from build123d import *

# Parameters (mm, degrees)
F0_W      = 609.6
F0_H      = 38.1
F1_DEPTH  = 203.2
F3_D      = 5.1054
F5_D      = 5.1054
F5_DEPTH  = 25.4
F5_TIP    = 1.5338169022
F7_D      = 5.1054
F7_DEPTH  = 25.4
F7_TIP    = 1.5338169022
F8_R      = 5.08
F9_DEPTH  = 7.62
F12_DEPTH = 38.101


# Not quite as in the source:
# - the program builds the solid bodies; features that only make, move or delete a surface that nothing else refers to are left out


with BuildPart() as f1:
    # F0 (on Front) → F1 (new body)
    with BuildSketch(Plane.XZ):
        with Locations((304.8, 19.05)):
            Rectangle(F0_W, F0_H)
    extrude(amount=-F1_DEPTH)

    # F3 (through all)
    with Locations(Plane.XY.offset(38.1)):
        with Locations((152.4, 157.950154), (177.8, 157.950154), (152.4, 45.249846), (177.8, 45.249846)):
            Hole(F3_D / 2)

    # F5
    with Locations(Plane.XZ):
        with Locations((228.6, 19.05), (241.3, 19.05), (254, 19.05), (266.7, 19.05), (279.4, 19.05), (292.1, 19.05), (304.8, 19.05), (317.5, 19.05), (330.2, 19.05), (342.9, 19.05), (355.6, 19.05), (368.3, 19.05), (381, 19.05), (393.7, 19.05), (406.4, 19.05), (419.1, 19.05), (431.8, 19.05), (444.5, 19.05), (457.2, 19.05), (469.9, 19.05), (482.6, 19.05), (495.3, 19.05), (508, 19.05), (520.7, 19.05)):
            Hole(F5_D / 2, depth=F5_DEPTH)
            with Locations((0, 0, -(F5_DEPTH + F5_TIP / 2))):  # 118° drill point
                Cone(0, F5_D / 2, F5_TIP, mode=Mode.SUBTRACT)

    # F7
    with Locations(Plane(origin=(0, 203.2, 0), x_dir=(-1, 0, 0), z_dir=(0, 1, 0))):
        with Locations((-228.6, 19.05), (-241.3, 19.05), (-254, 19.05), (-266.7, 19.05), (-279.4, 19.05), (-292.1, 19.05), (-304.8, 19.05), (-317.5, 19.05), (-330.2, 19.05), (-342.9, 19.05), (-355.6, 19.05), (-368.3, 19.05), (-381, 19.05), (-393.7, 19.05), (-406.4, 19.05), (-419.1, 19.05), (-431.8, 19.05), (-444.5, 19.05), (-457.2, 19.05), (-469.9, 19.05), (-482.6, 19.05), (-495.3, 19.05), (-508, 19.05), (-520.7, 19.05)):
            Hole(F7_D / 2, depth=F7_DEPTH)
            with Locations((0, 0, -(F7_DEPTH + F7_TIP / 2))):  # 118° drill point
                Cone(0, F7_D / 2, F7_TIP, mode=Mode.SUBTRACT)

    # F8 (on face) → F9 (cut)
    with BuildSketch(Plane(origin=(0, 0, 0), x_dir=(1, 0, 0), z_dir=(0, 0, -1))):
        with Locations((177.8, -157.950154)):
            Circle(F8_R)
        with Locations((152.4, -157.950154)):
            Circle(F8_R)
        with Locations((177.8, -45.249846)):
            Circle(F8_R)
        with Locations((152.4, -45.249846)):
            Circle(F8_R)
    extrude(amount=-F9_DEPTH, mode=Mode.SUBTRACT)

    # F11 (on face) → F12 (cut, through all)
    with BuildSketch(Plane(origin=(0, 0, 0), x_dir=(1, 0, 0), z_dir=(0, 0, -1))):
        with BuildLine():
            ThreePointArc((211.7379009724, -154.5971), (208.4740009724, -157.861), (211.7379009724, -161.1249))
            Line((211.7379009724, -161.1249), (491.1379009724, -161.1249))
            ThreePointArc((491.1379009724, -161.1249), (494.4018009724, -157.861), (491.1379009724, -154.5971))
            Line((491.1379009724, -154.5971), (211.7379009724, -154.5971))
        make_face()
        with BuildLine():
            ThreePointArc((211.7379009724, -42.0751), (208.4740009724, -45.339), (211.7379009724, -48.6029))
            Line((211.7379009724, -48.6029), (491.1379009724, -48.6029))
            ThreePointArc((491.1379009724, -48.6029), (494.4018009724, -45.339), (491.1379009724, -42.0751))
            Line((491.1379009724, -42.0751), (211.7379009724, -42.0751))
        make_face()
    extrude(amount=-F12_DEPTH, mode=Mode.SUBTRACT)


solid = f1.part
Could you check a few things on this model? Use its own coordinates, in mm. A direction names the side the tool comes from. Coordinates: 2 decimals unless noted, no trailing zeros. Order: outer loops, then holes, each group sorted by start corner. A loop starts at its lowest first (then second) coordinate and runs counter-clockwise, first axis right, second up. Notation, with made-up numbers: (3, 80) -> (7, 80) arc R18 ccw to (7, 113) -> close; hole circle Ø11 at (27.25, 73). An arc over 180 degrees is marked (long way). One line per item, written item: value. Start each with the question number.
1) If I drill on L1, parallel to Y at x = 414, z = 15; L2, parallel to Z at x = 495.3, y = 193; L3, parallel to Z at x = 266, y = 11, over which ranges is the centre line in solid material (lowest first)? Write a range as [from, to].
2) Imagine slicing it at B-B on y = 13.5. Count the separate pieces of the cut face and the enclosed holes in it, plus the area to 3 significant figures.
3) We'd pull the mould along X, two halves only. Please class faces 4 (the flat face through (301, 100, 0)), 5 (the flat face through (0, 100, 19)), 6 (the flat face through (349, 48.603, 19)): +X half, -X half, draft (parallel to the pull), parting line (faces both ways), or undercut.
4) Which directions (+Z, -Z, +X, -X, +Y, -Y) give clear straight access to the entire face, cutting with the end or side of a thin tool? Please do faces 1 (the flat face through (301, 100, 38.1)), 2 (the flat face through (353, 42.075, 19)), 3 (the cylindrical face through (173.77, 48.34, 3.76)).
5) Imagine slicing it at A-A on x = 219. List the corners of the cut face in (y, z) for me.
6) I'm going to push flat-ended pins straight in: pin 1 (4.5 mm diameter, centred on x = 444.5, z = 19.05, fed in from -Y); pin 2 (4 mm diameter, centred on x = 368.3, z = 19.05, fed in from +Y); pin 3 (4 mm diameter, centred on x = 495.3, z = 19.05, fed in from -Y). Where does each tip first touch, or does it pass through?
Answer list:
1. L1: y = [0, 42.08], [48.6, 154.6], [161.12, 203.2]
1. L2: z = [0, 16.5], [21.6, 38.1]
1. L3: z = [0, 16.6], [21.5, 38.1]
2. separate pieces: 1
2. enclosed holes: 24
2. area: 22,700 mm2
3. face 4: draft
3. face 5: -X half
3. face 6: undercut
4. face 1: +Z, +X, -X, +Y, -Y
4. face 2: +Z, -Z
4. face 3: -Z
5. outline: (0, 0) -> (42.08, 0) -> (42.08, 38.1) -> (0, 38.1) -> close; (48.6, 0) -> (154.6, 0) -> (154.6, 38.1) -> (48.6, 38.1) -> close; (161.12, 0) -> (203.2, 0) -> (203.2, 38.1) -> (161.12, 38.1) -> close
6. pin 1: stops at y = 25.58
6. pin 2: stops at y = 177.47
6. pin 3: stops at y = 25.73
